```python
from build123d import *

# Parameters (mm, degrees)
F1_DEPTH = 7
F2_R     = 1


with BuildPart() as f1:
    # F0 (on Front) → F1 (new body)
    with BuildSketch(Plane.XZ):
        with BuildLine():
            ThreePointArc((3.163336, 6.244462), (3.590379, 6.009091), (4, 5.744563))
            Line((4, 5.744563), (4, 9.744563))
            Line((4, 9.744563), (-4, 9.744563))
            Line((-4, 9.744563), (-4, 5.744563))
            ThreePointArc((-4, 5.744563), (-3.590379, 6.009091), (-3.163336, 6.244462))
            Line((-3.163336, 6.244462), (-3.65142, 7.340716))
            Line((-3.65142, 7.340716), (-3.011938, 7.625432))
            Line((-3.011938, 7.625432), (-2.045407, 7.939477))
            Line((-2.045407, 7.939477), (-1.360704, 8.085015))
            Line((-1.360704, 8.085015), (-0.35, 8.191245))
            Line((-0.35, 8.191245), (0.35, 8.191245))
            Line((0.35, 8.191245), (1.360704, 8.085015))
            Line((1.360704, 8.085015), (2.045407, 7.939477))
            Line((2.045407, 7.939477), (2.971265, 7.534078))
            Line((2.971265, 7.534078), (3.610747, 7.249362))
            Line((3.610747, 7.249362), (3.163336, 6.244462))
        make_face()
    extrude(amount=F1_DEPTH)

    # F2
    f2_edges = [f1.edges().sort_by_distance(p)[0] for p in [
        (-4, -7, 7.744563),
        (4, -7, 7.744563),
        (4, 0, 7.744563),
        (-4, 0, 7.744563),
        (4, -3.5, 9.744563),
        (-4, -3.5, 9.744563),
        (0, 0, 9.744563),
        (0, -7, 9.744563),
    ]]
    fillet(f2_edges, radius=F2_R)


solid = f1.part
```
Could you check a few things on this model? Use its own coordinates, in mm. A direction names the side the tool comes from. Round coordinates to 2 decimals unless told otherwise and drop trailing zeros. Write each loop counter-clockwise with the first axis right and the second up, starting at its lowest first coordinate (ties: lowest second). Pieces come first, ordered by that corner, then holes.
(1) Suppose I cut it at B-B on y = -2.25. Write out the boundary of the cut face in (x, z).
Findings below:
outline: (-4, 5.74) arc R7 cw to (-3.16, 6.24) - (-3.65, 7.34) - (-3.01, 7.63) - (-2.05, 7.94) - (-1.36, 8.09) - (-0.35, 8.19) - (0.35, 8.19) - (1.36, 8.09) - (2.05, 7.94) - (2.97, 7.53) - (3.61, 7.25) - (3.16, 6.24) arc R7 cw to (4, 5.74) - (4, 8.74) arc R1 ccw to (3, 9.74) - (-3, 9.74) arc R1 ccw to (-4, 8.74) - close
(2) Suppose I cut it at D-D on x = -1.25. Write out the boundary of the cut face in (y, z), and give its area (3 significant figures).
Findings below:
outline: (-7, 8.1) - (0, 8.1) - (0, 8.74) arc R1 ccw to (-1, 9.74) - (-6, 9.74) arc R1 ccw to (-7, 8.74) - close
area: 11.1 mm2
(3) Suppose I cut it at C-C on x = -0.25. Write out the boundary of the cut face in (y, z).
Findings below:
outline: (-7, 8.19) - (0, 8.19) - (0, 8.74) arc R1 ccw to (-1, 9.74) - (-6, 9.74) arc R1 ccw to (-7, 8.74) - close
(4) For pin 1 (1.5 mm diameter, centred on x = -0.5, y = -5.5, fed in from -Z), with a flat end and sliding along its axis, tell me the tip position at first contact or that it passes through.
Findings below:
pin 1: stops at z = 8.1
(5) If I drill on probe 1 along Z at (x, y) = (-3.25, -1.5); probe 2 along X at (y, z) = (-3.5, 7.4); probe 3 along X at (y, z) = (-0.5, 7.1), over which ranges is the centre line in solid material (lowest first)?
Findings below:
probe 1: z = 6.2 to 6.44, 7.52 to 9.71
probe 2: x = -4 to -3.52, 3.27 to 4
probe 3: x = -3.87 to -3.54, 3.54 to 3.87
(6) Which directions (+Z, -Z, +X, -X, +Y, -Y) give clear straight access to the entire face, cutting with the end or side of a thin tool? Please do faces 1 (the face through (-3.4, -3.45, 6.78)), 2 (the face through (3.8, -6.6, 7.3)), 3 (the face through (0.85, -3.45, 8.14)).
Findings below:
face 1: +Y, -Y
face 2: +Z, -Z, +X, -Y
face 3: -Z, +Y, -Y
(7) Thinking about a two-plate mould opening in X: for faces 4 (the face through (-3.8, -0.4, 7.2)), 5 (the face through (4, -3, 7)), 6 (the face through (0, -3, 9.745)), 7 (the face through (3.39, -3.45, 6.75)), which applies, +X half, -X half, draft (parallel to the pull), parting line (faces both ways), or undercut?
Findings below:
face 4: -X half
face 5: +X half
face 6: draft
face 7: undercut
(8) Suppose I cut it at A-A on z = 6.4. Write out the boundary of the cut face in (x, y).
Findings below:
outline: (-4, -6) arc R1 ccw to (-3.23, -6.97) - (-3.23, -0.03) arc R1 ccw to (-4, -1) - close; (3.23, -6.97) arc R1 ccw to (4, -6) - (4, -1) arc R1 ccw to (3.23, -0.03) - close
